from build123d import *

# Parameters (mm, degrees)
F0_W      = 31.7881
F0_H      = 15.8369
F1_DEPTH  = 4.7879
F2_R      = 2.4511
F3_DEPTH  = 1.778
F4_R      = 2.4511
F5_DEPTH  = 1.778
F6_R      = 2.4511
F7_DEPTH  = 1.778
F8_R      = 2.4511
F9_DEPTH  = 1.778
F10_R     = 2.4511
F11_DEPTH = 1.778
F12_R     = 2.4511
F13_DEPTH = 1.778
F14_R     = 2.4511
F15_DEPTH = 1.778
F16_R     = 2.4511
F17_DEPTH = 1.778
F20_R     = 2.82575
F22_DEPTH = 8.3185
F20_W     = 30.5308
F20_H     = 14.5796
F20_R_2   = 3.2385
F23_DEPTH = 8.3185
F24_R     = 3.2385
F28_DEPTH = 8.3312
F25_R     = 3.2385
F29_DEPTH = 8.3312
F26_R     = 2.8194
F30_DEPTH = 8.3312
F27_R     = 2.8194
F31_DEPTH = 8.3312


# Not quite as in the source:
# - the program builds the solid bodies; features that only make, move or delete a surface that nothing else refers to are left out


with BuildPart() as f1:
    # F0 (on Top) → F1 (new body, symmetric)
    with BuildSketch(Plane.XY):
        Rectangle(F0_W, F0_H)
    extrude(amount=F1_DEPTH, both=True)

    # F2 (on face) → F3 (join)
    with BuildSketch(Plane.XY.offset(4.7879)):
        with Locations((-11.91895, 3.98145)):
            Circle(F2_R)
    extrude(amount=F3_DEPTH)

    # F4 (on face) → F5 (join)
    with BuildSketch(Plane.XY.offset(4.7879)):
        with Locations((-3.9052600634, 3.96875)):
            Circle(F4_R)
    extrude(amount=F5_DEPTH)

    # F6 (on face) → F7 (join)
    with BuildSketch(Plane.XY.offset(4.7879)):
        with Locations((4.0955786651, 3.91795)):
            Circle(F6_R)
    extrude(amount=F7_DEPTH)

    # F8 (on face) → F9 (join)
    with BuildSketch(Plane.XY.offset(4.7879)):
        with Locations((12.096326677, 3.98145)):
            Circle(F8_R)
    extrude(amount=F9_DEPTH)

    # F10 (on face) → F11 (join)
    with BuildSketch(Plane.XY.offset(4.7879)):
        with Locations((-11.89355, -3.96875)):
            Circle(F10_R)
    extrude(amount=F11_DEPTH)

    # F12 (on face) → F13 (join)
    with BuildSketch(Plane.XY.offset(4.7879)):
        with Locations((-3.86715, -3.96875)):
            Circle(F12_R)
    extrude(amount=F13_DEPTH)

    # F14 (on face) → F15 (join)
    with BuildSketch(Plane.XY.offset(4.7879)):
        with Locations((4.15925, -3.96875)):
            Circle(F14_R)
    extrude(amount=F15_DEPTH)

    # F16 (on face) → F17 (join)
    with BuildSketch(Plane.XY.offset(4.7879)):
        with Locations((11.91895, -3.96875)):
            Circle(F16_R)
    extrude(amount=F17_DEPTH)

    # F20 (on face) → F22 (cut)
    with BuildSketch(Plane(origin=(0, 0, -4.7879), x_dir=(1, 0, 0), z_dir=(0, 0, -1))):
        Circle(F20_R)
    extrude(amount=-F22_DEPTH, mode=Mode.SUBTRACT)

    # F20 (on face) → F23 (cut)
    with BuildSketch(Plane(origin=(0, 0, -4.7879), x_dir=(1, 0, 0), z_dir=(0, 0, -1))):
        Rectangle(F20_W, F20_H)
        Circle(F20_R_2, mode=Mode.SUBTRACT)
    extrude(amount=-F23_DEPTH, mode=Mode.SUBTRACT)

    # F24 (on face) → F28 (join)
    with BuildSketch(Plane(origin=(0, 0, -4.7879), x_dir=(1, 0, 0), z_dir=(0, 0, -1))):
        with Locations((-8.4963, 0)):
            Circle(F24_R)
    extrude(amount=-F28_DEPTH)

    # F25 (on face) → F29 (join)
    with BuildSketch(Plane(origin=(0, 0, -4.7879), x_dir=(1, 0, 0), z_dir=(0, 0, -1))):
        with Locations((8.4963, 0)):
            Circle(F25_R)
    extrude(amount=-F29_DEPTH)

    # F26 (on face) → F30 (cut)
    with BuildSketch(Plane(origin=(0, 0, -4.7879), x_dir=(1, 0, 0), z_dir=(0, 0, -1))):
        with Locations((-8.472575021, 0)):
            Circle(F26_R)
    extrude(amount=-F30_DEPTH, mode=Mode.SUBTRACT)

    # F27 (on face) → F31 (cut)
    with BuildSketch(Plane(origin=(0, 0, -4.7879), x_dir=(1, 0, 0), z_dir=(0, 0, -1))):
        with Locations((8.4932660684, 0)):
            Circle(F27_R)
    extrude(amount=-F31_DEPTH, mode=Mode.SUBTRACT)


solid = f1.part
CAD build for the part. Positions are in the model's coordinates, mm. A direction names the side the tool comes from. Round coordinates to 2 decimals unless told otherwise and drop trailing zeros. Order: outer loops, then holes, each group sorted by start corner. A loop starts at its lowest first (then second) coordinate and runs counter-clockwise, first axis right, second up. Notation, with made-up numbers: (-4.75, -38.5) -> (16.25, -38.5) arc R13 ccw to (16.25, -15.5) -> close; hole circle Ø10 at (7, -19.75). An arc over 180 degrees is marked (long way). Write item = value, one per line. Start each with the question number.
(1) Pin check, flat tips, straight feed: P1, Ø7.5, axis at x = 8.49, y = 0, coming from the +Z side; P2, Ø1, axis at x = -1, y = 2, coming from the -Z side; P3, Ø4.5, axis at x = 0, y = 0, coming from the +Z side. Stop position of each tip, or through.
(2) Which spindle directions (+Z, -Z, +X, -X, +Y, -Y) get a long thin tool onto all of the face, cutting with end or side? Do faces 4 (the flat face through (0, 7.29, -1)), 5 (the cylindrical face through (-13.84, -5.46, 5.66)), 6 (the flat face through (4, 4, 6.566)). Say none if no direction does.
(3) Cut at D-D, the plane x = 10. List the corners of the cut face in (y, z).
(4) Cut at A-A, the plane z = -1. List the corners of the cut face in (x, y).
(5) Pull direction X, two halves, no side cores. Call faces 1 (the flat face through (0, 0, 4.788)), 2 (the flat face through (15.894, 0, 0)), 3 (the flat face through (12, -4, 6.566)): released by +X, released by -X, zero draft, split by the parting line, or undercut.
(6) Cut at B-B, the plane x = 0. List the corners of the cut face in (y, z), then the cut area to 3 significant figures.
(7) Probe line 1 (Y direction, x = 0, z = -0.75); line 2 (Y direction, x = 12, z = 1.5); line 3 (Y direction, x = 2.5, z = -3.75). List the from-to ranges inside material, lowest first. Write a range as [from, to].
Model answer:
q1.P1 = 6.57
q1.P2 = 3.53
q1.P3 = 4.79
q2.face_4 = -Z
q2.face_5 = +Z
q2.face_6 = +Z, +X, -X, +Y, -Y
q3.outline = (-7.92, -4.79) -> (-7.29, -4.79) -> (-7.29, 3.53) -> (-2.87, 3.53) -> (-2.87, -4.79) -> (-2.38, -4.79) -> (-2.38, 3.54) -> (2.38, 3.54) -> (2.38, -4.79) -> (2.87, -4.79) -> (2.87, 3.53) -> (7.29, 3.53) -> (7.29, -4.79) -> (7.92, -4.79) -> (7.92, 4.79) -> (5.25, 4.79) -> (5.25, 6.57) -> (2.71, 6.57) -> (2.71, 4.79) -> (-2.44, 4.79) -> (-2.44, 6.57) -> (-5.49, 6.57) -> (-5.49, 4.79) -> (-7.92, 4.79) -> close
q4.outline = (-15.89, -7.92) -> (15.89, -7.92) -> (15.89, 7.92) -> (-15.89, 7.92) -> close; circle Ø6.48 at (-8.5, 0); circle Ø6.48 at (0, 0); circle Ø6.48 at (8.5, 0); hole (-15.27, -7.29) -> (15.27, -7.29) -> (15.27, 7.29) -> (-15.27, 7.29) -> close; hole circle Ø5.64 at (-8.47, 0); hole circle Ø5.65 at (0, 0); hole circle Ø5.64 at (8.49, 0)
q5.face_1 = undercut
q5.face_2 = released by +X
q5.face_3 = zero draft
q6.outline = (-7.92, -4.79) -> (-7.29, -4.79) -> (-7.29, 3.53) -> (-3.24, 3.53) -> (-3.24, -4.79) -> (-2.83, -4.79) -> (-2.83, 3.53) -> (2.83, 3.53) -> (2.83, -4.79) -> (3.24, -4.79) -> (3.24, 3.53) -> (7.29, 3.53) -> (7.29, -4.79) -> (7.92, -4.79) -> (7.92, 4.79) -> (-7.92, 4.79) -> close
q6.area = 37.2 mm2
q7.line_1 = [-7.92, -7.29], [-3.24, -2.83], [2.83, 3.24], [7.29, 7.92]
q7.line_2 = [-7.92, -7.29], [7.29, 7.92]
q7.line_3 = [-7.92, -7.29], [-2.06, -1.32], [1.32, 2.06], [7.29, 7.92]
